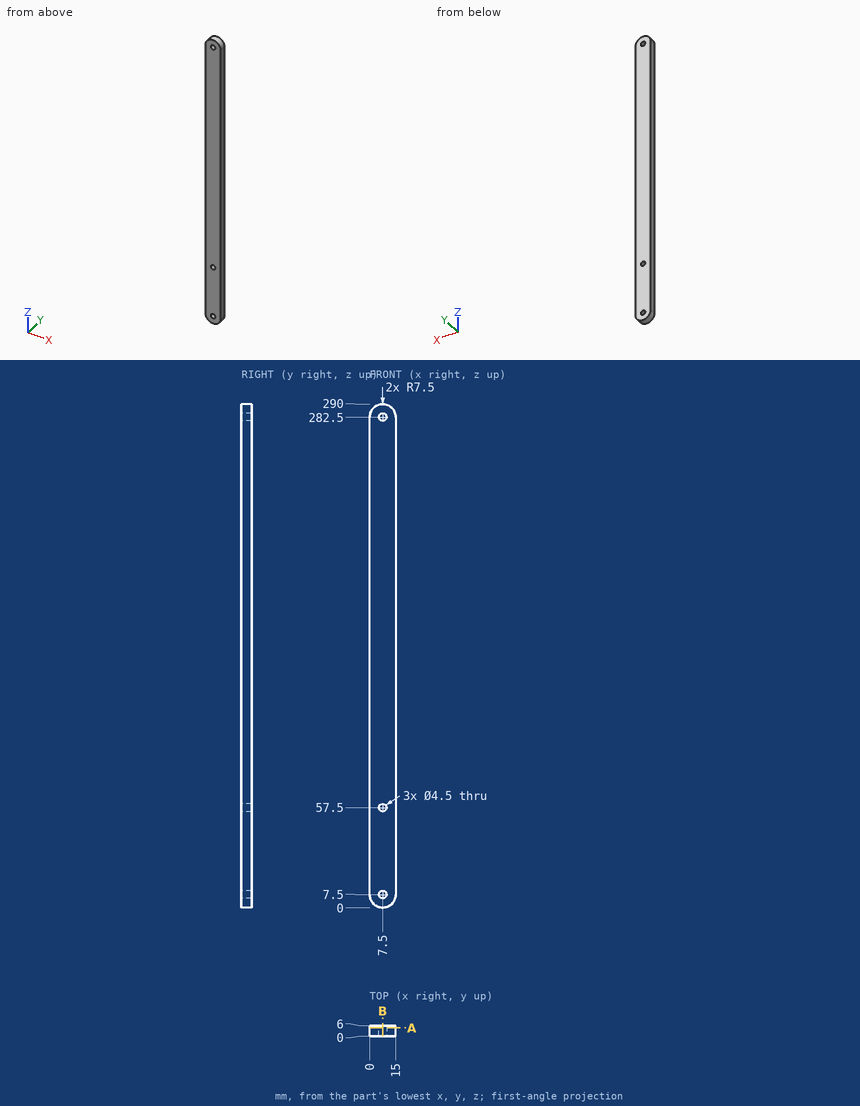
Drawing for the job (mm, zero at the part's lowest x, y, z). Round coordinates to 2 decimals unless told otherwise and drop trailing zeros. Loops run counter-clockwise (first coordinate to the right, second up) from the corner with the lowest first, then second, coordinate; pieces in that order, holes last. Notation, with made-up numbers: (18, 44) -> (32, 44) arc R26 ccw to (32, 63) -> close; hole circle Ø9 at (-18, -7). An arc over 180 degrees is marked (long way). Use one line per item in the form item = value. Start each with the question number.
Item 1: Band-saw the part on B-B (x = 7.5). List the corners of the cut face in (y, z), plus the area to 3 significant figures.
Item 2: Drill centre lines: line 1 along Z through (x, y) = (7.5, 4); line 2 along Z through (x, y) = (5.5, 3.55); line 3 along X through (y, z) = (4.2, 282.5). Where is each one in solid material? Low to high.
Item 3: Drop flat-ended pins along their axis: pin 1 Ø3 at (x, y) = (3.5, 3.5) entering from +Z; pin 2 Ø3.5 at (x, z) = (7.5, 282.5) entering from -Y; pin 3 Ø3 at (x, y) = (3, 2.5) entering from +Z. Give the stop position or say it passes through.
Item 4: Band-saw the part on A-A (y = 4.7). List the corners of the cut face in (x, z), plus the area to 3 significant figures.
Data:
q1.outline = (0, 0) -> (6, 0) -> (6, 5.25) -> (0, 5.25) -> close; (0, 9.75) -> (6, 9.75) -> (6, 55.25) -> (0, 55.25) -> close; (0, 59.75) -> (6, 59.75) -> (6, 280.25) -> (0, 280.25) -> close; (0, 284.75) -> (6, 284.75) -> (6, 290) -> (0, 290) -> close
q1.area = 1,660 mm^2
q2.line_1 = 0 to 5.25, 9.75 to 55.25, 59.75 to 280.25, 284.75 to 290
q2.line_2 = 0.27 to 6.47, 8.53 to 56.47, 58.53 to 281.47, 283.53 to 289.73
q2.line_3 = 0 to 5.25, 9.75 to 15
q3.pin_1 = 289.57
q3.pin_2 = through
q3.pin_3 = 289.37
q4.outline = (0, 7.5) arc R7.5 ccw to (15, 7.5) -> (15, 282.5) arc R7.5 ccw to (0, 282.5) -> close; hole circle Ø4.5 at (7.5, 7.5); hole circle Ø4.5 at (7.5, 57.5); hole circle Ø4.5 at (7.5, 282.5)
q4.area = 4,250 mm^2
